For this review, take the finished solid that the model builds, in its own axes (mm). Face numbers are marked on the shaded views. A direction names the side the tool comes from. Give positions to 0.01 mm unless a question says otherwise; leave off trailing zeros. Order: outer loops, then holes, each group sorted by start corner. A loop starts at its lowest first (then second) coordinate and runs counter-clockwise, first axis right, second up. Notation, with made-up numbers: (80, 79.25) - (86, 79.25) arc R25 cw to (86, 104.25) - close; hole circle Ø5 at (47, -22). An arc over 180 degrees is marked (long way). Use a Markdown table: item, result. Add a question column.
1) Wall thickness on L1, parallel to X at y = 16, z = -3; L2, parallel to Z at x = 5.25, y = 12.7; L3, parallel to Y at x = 0.5, z = -21: over which ranges is each line inside the solid? List them lowest first.
2) We need section C-C on z = -4. Write out the cut boundary in (x, y).
3) We need section D-D on x = -9. Write out the cut boundary in (y, z).
4) Clearance check with flat-ended pins moving along their axes: P1, Ø5, axis at x = 2.5, z = 9, coming from the +Y side; P2, Ø7.5, axis at x = -17, z = -26.5, coming from the -Y side; P3, Ø4, axis at x = -4.5, y = 12.5, coming from the +Z side. State where each tip first meets the part, or that it passes through.
5) We need section A-A on x = -12.7. Write out the cut boundary in (y, z).
6) Machinability: for the marked faces 1, 2 and 3, which of the approach directions +Z, -Z, +X, -X, +Y, -Y give a long, thin tool a straight path to every point of the face, cutting with its end or side? Answer none if there is none.
7) We need section B-B on y = 12. Write out the cut boundary in (x, z), then the cut area to 3 significant figures.
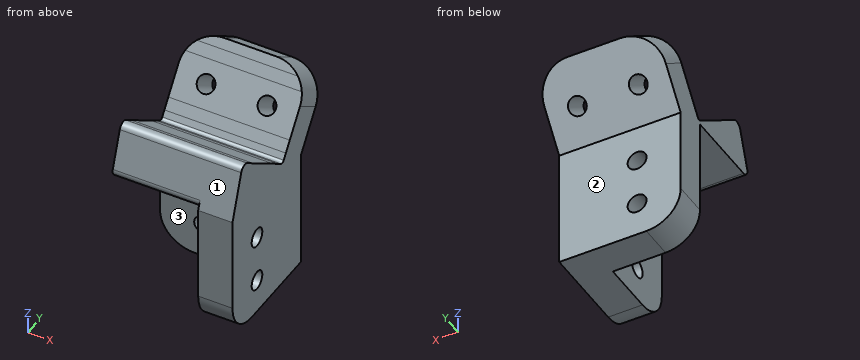
Autodesk Inventor part; units mm, degrees
ref_plane "YZ Plane" through (0, 0, 0) normal (1, 0, 0) x (0, 1, 0)
ref_plane "XZ Plane" through (0, 0, 0) normal (0, 1, 0) x (-1, 0, 0)
ref_plane "XY Plane" through (0, 0, 0) normal (0, 0, 1) x (1, 0, 0)
sketch "Sketch1" plane through (0, 0, 0) normal (1, 0, 0) x (0, 1, 0)
  line L0 (0, 0) -> (25.4, 0)
  line L1 (25.4, 0) -> (25.4, -38.1)
  line L2 (25.4, -38.1) -> (0, -38.1)
  line L3 (0, -38.1) -> (0, 0)
  circle A0 centre (12.7, -27.9675) radius 2.75
  circle A1 centre (12.7, -13.8886) radius 2.75
  dimension "d0" = 25.4
  dimension "d1" = 38.1
  dimension "d2" = 5.5
extrude "Extrusion1" add sketch "Sketch1" along normal blind 10
sketch "Sketch2" plane through (10, 0, 0) normal (1, 0, 0) x (0, 0, -1)
  line L0 (-11.9576, 10.5414) -> (-13.9859, 7.7441)
  line L1 (-2.4758, 23.6177) -> (-4.5041, 20.8204)
  line L2 (-18.0308, 7.0996) -> (-20.828, 9.1279)
  line L3 (-31.1071, 16.5813) -> (-33.9043, 18.6096)
  line L4 (-34.5489, 22.6546) -> (-32.5206, 25.4518)
  line L5 (-25.0672, 35.7309) -> (-23.0389, 38.5281)
  line L6 (-3.1204, 27.6626) -> (-5.9176, 29.6909)
  line L7 (-16.1967, 37.1443) -> (-18.9939, 39.1726)
  line L8 (38.1, 0) -> (38.1, 25.4)
  line L9 (38.1, 25.4) -> (0, 25.4)
  line L10 (0, 25.4) -> (0, 0)
  line L11 (0, 0) -> (38.1, 0)
  circle A0 centre (13.8886, 12.7) radius 2.75
  circle A1 centre (27.9675, 12.7) radius 2.75
  line L12 (-0.7756, 25.9624) -> (-21.3387, 40.8728)
  line L13 (-0.7756, 25.9624) -> (0, 25.4)
  line L14 (-15.6861, 5.3994) -> (-0.7756, 25.9624)
  line L15 (-15.6861, 5.3994) -> (0, 0)
  line L16 (-15.6861, 5.3994) -> (-36.2491, 20.3098)
  line L17 (-21.3387, 40.8728) -> (-15.4684, 48.9685)
  line L18 (-15.4684, 48.9685) -> (17.7637, 24.8716)
  line L19 (17.7637, 24.8716) -> (11.8935, 16.7759)
  line L20 (11.8935, 16.7759) -> (-21.3387, 40.8728)
  line L21 (-15.6861, 5.3994) -> (-36.2491, 20.3098)
  line L22 (38.1, 0) -> (0, 0)
  line L23 (38.1, 25.4) -> (38.1, 35.4)
  line L24 (38.1, 35.4) -> (1.1477, 35.4)
  line L25 (1.1477, 35.4) -> (1.1477, 25.4)
  line L26 (1.1477, 25.4) -> (38.1, 25.4)
  point P0 (17.035, 25.4)
  point P1 (3.244, 35.4)
  dimension "d5" = 10
  dimension "d10" = 10
extrude "Extrusion2" add sketch "Sketch2" against normal blind 35.4 contours L14 L1 L13 L10 L15 L0 | L12 L6 L7 L17 L18 L24 L25 L9 L13 | L25 L24 L18 L9 | L9 L18 L24 L23
sketch "Sketch3" plane through (0, 25.4, -38.1) normal (0, -1, 0) x (1, 0, 0)
  line L0 (0, 0) -> (0, 38.1)
  line L1 (0, 38.1) -> (-25.4, 38.1)
  line L2 (-25.4, 0) -> (-25.4, 38.1)
  line L3 (0, 0) -> (-25.4, 0)
  line L4 (10, 12.8825) -> (10, 7.3825)
  line L5 (0, 12.8825) -> (0, 7.3825)
  line L6 (10, 26.9614) -> (10, 21.4614)
  circle A0 centre (-12.7, 10.1325) radius 2.75
  circle A1 centre (-12.7, 24.2114) radius 2.75
  point P0 (0, 38.1)
extrude "Extrusion3" cut sketch "Sketch3" against normal blind 35.4 contours A0 | A1
sketch "Sketch4" plane through (-25.4, 40.8728, 21.3387) normal (0, -0.8096, 0.587) x (1, 0, 0)
  line L0 (35.4, 0) -> (35.4, -25.4)
  line L1 (35.4, 0) -> (0, 0)
  line L2 (0, -25.4) -> (0, 0)
  line L3 (35.4, -25.4) -> (0, -25.4)
  line L4 (26.667, -12.7) -> (8.9084, -12.7) construction
  line L5 (26.667, -10.1) -> (8.9084, -10.1)
  line L6 (8.9084, -15.3) -> (26.667, -15.3)
  arc A0 (26.667, -15.3) -> (26.667, -10.1) centre (26.667, -12.7) ccw
  arc A1 (8.9084, -10.1) -> (8.9084, -15.3) centre (8.9084, -12.7) ccw
  circle A2 centre (26.667, -12.7) radius 2.6
  circle A3 centre (8.9084, -12.7) radius 2.6
  point P0 (25.4, -41.2685)
  point P1 (17.7877, -12.7)
  point P2 (8.9084, -10.1)
  point P3 (26.667, -10.1)
  dimension "d13" = 2.6
extrude "Extrusion4" cut sketch "Sketch4" against normal blind 35.4 contours A0 A2 | A3 A1
fillet "Fillet1" radius 10 4 edges at (5, 0, -38.1) (-25.4, 30.4, -38.1) (10, 44.9207, 18.4035) (-25.4, 44.9207, 18.4035)
fillet "Fillet2" radius 2 2 edges at (-12.7, 0, 0) (-7.7, 5.3994, 15.6861)
fillet "Fillet3" radius 1 1 edges at (-7.7, 25.9624, 0.7756)
properties part number "upperRearBracket"
Checked values:
| question | item | result |
|---|---|---|
| 1 | L1 | 0 to 10 |
| 1 | L2 | -38.1 to -30.72, -25.22 to -16.64, -11.14 to 10.39 |
| 1 | L3 | 0 to 35.4 |
| 2 | outline | (-25.4, 25.4) - (0, 25.4) - (0, 0) - (10, 0) - (10, 35.4) - (-25.4, 35.4) - close |
| 3 | outline | (0.91, 2.65) arc R2 ccw to (2.8, 0) - (25.4, 0) - (25.4, -38.1) - (35.4, -38.1) - (35.4, -3.24) - (48.97, 15.47) - (40.87, 21.34) - (39.17, 18.99) - (37.14, 16.2) - (29.69, 5.92) - (27.66, 3.12) - (26.55, 1.59) arc R1 cw to (25.15, 1.36) - (23.62, 2.48) - (20.82, 4.5) - (10.54, 11.96) - (7.74, 13.99) - (7.59, 14.1) arc R2 ccw to (4.52, 13.13) - close |
| 4 | P1 | y = 46.09 |
| 4 | P2 | y = 25.4 |
| 4 | P3 | z = 11.99 |
| 5 | outline | (0.91, 2.65) arc R2 ccw to (2.8, 0) - (25.4, 0) - (25.4, -11.14) - (35.4, -11.14) - (35.4, -3.24) - (48.97, 15.47) - (40.87, 21.34) - (39.17, 18.99) - (37.14, 16.2) - (29.69, 5.92) - (27.66, 3.12) - (26.55, 1.59) arc R1 cw to (25.15, 1.36) - (23.62, 2.48) - (20.82, 4.5) - (10.54, 11.96) - (7.74, 13.99) - (7.59, 14.1) arc R2 ccw to (4.52, 13.13) - close; (25.4, -38.1) - (35.4, -38.1) - (35.4, -30.72) - (25.4, -30.72) - close; (25.4, -25.22) - (35.4, -25.22) - (35.4, -16.64) - (25.4, -16.64) - close |
| 6 | face 1 | +Z, +X, -X, -Y |
| 6 | face 2 | -Z, +X, -X, +Y |
| 6 | face 3 | -Z, -X, -Y |
| 7 | outline | (-25.4, 0) - (0, 0) - (0, -11.23) - (10, -11.23) - (10, 10.9) - (-25.4, 10.9) - close; (0, -38.1) - (10, -38.1) - (10, -30.63) - (0, -30.63) - close; (0, -25.31) - (10, -25.31) - (10, -16.55) - (0, -16.55) - close |
| 7 | area | 660 mm² |
